from build123d import *

# Parameters (mm, degrees)
F2_R     = 19.05
F3_DEPTH = 127
F4_SIZE  = 19.05


with BuildPart() as f1:
    # F0 (on Front) → F1 (revolve)
    with BuildSketch(Plane.XZ):
        with BuildLine():
            Line((0, -63.5), (0, 63.5))
            ThreePointArc((0, 63.5), (-63.5, 0), (0, -63.5))
        make_face()
    revolve(axis=Axis((0, 0, 0), (0, 0, -1)))

    # F2 (on Top) → F3 (join)
    with BuildSketch(Plane.XY):
        Circle(F2_R)
    extrude(amount=-F3_DEPTH)

    # F4
    f4_edges = [f1.edges().sort_by_distance(p)[0] for p in [
        (-19.05, 0, -127),
    ]]
    chamfer(f4_edges, length=F4_SIZE)


solid = f1.part
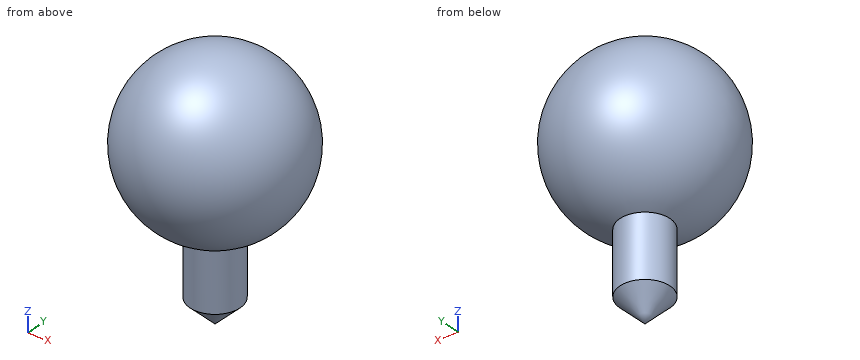
The listing builds one solid part. Answer for the finished solid, in the listing's coordinates (mm). Coordinates: 2 decimals unless noted, no trailing zeros. Write each loop counter-clockwise with the first axis right and the second up, starting at its lowest first coordinate (ties: lowest second). Pieces come first, ordered by that corner, then holes. Notation, with made-up numbers: (84.25, -11) - (104.25, -11) arc R27 cw to (104.25, 7) - close; hole circle Ø4 at (54.5, 31.5). An arc over 180 degrees is marked (long way). Return JSON: item names as keys, results as strings.
1. Each of these flat-tipped pins is pushed along its axis until it touches: pin 1 Ø3 at (y, z) = (-29, -59) entering from +X; pin 2 Ø3 at (y, z) = (14, -2) entering from +X; pin 3 Ø5 at (y, z) = (26, 41.5) entering from -X; pin 4 Ø2 at (y, z) = (-29.5, 14) entering from -X. Where does it stop, or does it pass through?
Final values:
{"pin 1": "through", "pin 2": "x = 62.23", "pin 3": "x = -43.27", "pin 4": "x = -55.05"}
2. The part is cut by section A-A on z = -105. Determine the outline of the cut face in (x, y), then the cut area to 3 significant figures.
Final values:
{"outline": "circle Ø38.1 at (0, 0)", "area": "1,140 mm^2"}
3. The part is cut by section B-B on x = -49. Determine the outline of the cut face in (y, z), then the cut area to 3 significant figures.
Final values:
{"outline": "circle Ø80.78 at (0, 0)", "area": "5,120 mm^2"}
4. Consider line 1 along Z through (x, y) = (-9, -58); line 2 along Y through (x, z) = (6.5, 51.5); line 3 along Z through (x, y) = (11, 23). Determine where each line is inside the solid, lowest interval first.
Final values:
{"line 1": "-24.23 to 24.23", "line 2": "-36.58 to 36.58", "line 3": "-58.16 to 58.16"}
